from build123d import *

# Parameters (mm, degrees)
SKETCH_1_W      = 36.5
SKETCH_1_H      = 22
EXTRUDE_1_DEPTH = 19
SKETCH_3_R      = 3
EXTRUDE_3_DEPTH = 20
FILLET_1_R      = 5
SKETCH_4_R      = 9
EXTRUDE_4_DEPTH = 24
FILLET_2_R      = 5


with BuildPart() as part:
    # 草图1 → 凸台-拉伸1 (new body)
    with BuildSketch(Plane(origin=(0, 0, 0), x_dir=(0, 0, -1), z_dir=(1, 0, 0))):
        with Locations((18.25, 11)):
            Rectangle(SKETCH_1_W, SKETCH_1_H)
    extrude(amount=EXTRUDE_1_DEPTH)

    # 草图3 → 凸台-拉伸3 (add, symmetric)
    with BuildSketch(Plane(origin=(9.5, 0, 0), x_dir=(0, 0, -1), z_dir=(1, 0, 0))):
        with Locations((25.5, 11)):
            Circle(SKETCH_3_R)
    extrude(amount=EXTRUDE_3_DEPTH, both=True)

    # 圆角1
    fillet_1_edges = [part.edges().sort_by_distance(p)[0] for p in [
        (9.5, 22, -36.5),
        (9.5, 0, -36.5),
    ]]
    fillet(fillet_1_edges, radius=FILLET_1_R)

    # 草图4 → 凸台-拉伸4 (add)
    with BuildSketch(Plane.XY):
        with Locations((9.5, 11.405533056)):
            Circle(SKETCH_4_R)
    extrude(amount=EXTRUDE_4_DEPTH)

    # 圆角2
    fillet_2_edges = [part.edges().sort_by_distance(p)[0] for p in [
        (0.5, 11.405533056, 24),
    ]]
    fillet(fillet_2_edges, radius=FILLET_2_R)


solid = part.part
Design review of the part built by this model. Coordinates are the model's own, in mm. A direction names the side the tool comes from. Round coordinates to 2 decimals unless told otherwise and drop trailing zeros. Loops run counter-clockwise (first coordinate to the right, second up) from the corner with the lowest first, then second, coordinate; pieces in that order, holes last. Notation, with made-up numbers: (41.25, 82.25) - (47.25, 82.25) arc R22 ccw to (47.25, 112.25) - close; hole circle Ø1 at (74, -14.5). An arc over 180 degrees is marked (long way). One line per item, written item: value. Start each with the question number.
1) Consider section B-B on x = 25. Give the boundary of the cut face in (y, z).
2) Draft analysis for pull direction X (two halves, no side actions). For faces 1 (the flat face through (29.5, 11, -25)), 2 (the flat face through (-10.5, 11, -25)), 3 (the cylindrical face through (14.338, 18.994, 9.367)), 4 (the flat face through (9, 11, -36.5)), state which applies: +X half, -X half, draft (parallel to the pull), parting line (faces both ways), or undercut.
3) Insertion check: pin 1 Ø8 at (x, z) = (17.5, 7) entering from -Y; pin 2 Ø1 at (y, z) = (4.5, -7) entering from +X; pin 3 Ø4 at (y, z) = (7, 18) entering from +X. Each pin has a flat end and moves straight along its axis. Give the tip position at first contact, or say it passes through.
4) Consider section C-C on z = -15. Give the boundary of the cut face in (x, y), then the cut area to 3 significant figures.
5) To check wall thickness, follow L1, parallel to X at y = 17.75, z = -7.5; L2, parallel to Z at x = -1, y = 10.75; L3, parallel to Z at x = 8, y = 7.5. State the ranges of each line that lie inside material, in increasing order. Write a range as from..to.
6) Consider section A-A on z = -25.5. Give the boundary of the cut face in (x, y), then the cut area to 3 significant figures.
7) For faces 5 (the cylindrical face through (24.3, 11.1, -22.5)), 6 (the cylindrical face through (-5.2, 11.1, -22.5)), 7 (the cylindrical face through (9.63, 1.43, -35)), 8 (the flat face through (1, 8, 0)), list the 3-axis set-ups (+Z, -Z, +X, -X, +Y, -Y) from which the entire face can be reached by the end or side of a thin tool; tool diameter is ignored.
Reported:
1. outline: circle Ø6 at (11, -25.5)
2. face 1: +X half
2. face 2: -X half
2. face 3: parting line
2. face 4: draft
3. pin 1: stops at y = 3.34
3. pin 2: stops at x = 19
3. pin 3: stops at x = 18.17
4. outline: (0, 0) - (19, 0) - (19, 22) - (0, 22) - close
4. area: 418 mm^2
5. L1: x = 0..19
5. L2: z = -28.49..-22.51
5. L3: z = -36.5..24
6. outline: (-10.5, 8) - (0, 8) - (0, 0) - (19, 0) - (19, 8) - (29.5, 8) - (29.5, 14) - (19, 14) - (19, 22) - (0, 22) - (0, 14) - (-10.5, 14) - close
6. area: 544 mm^2
7. face 5: +X
7. face 6: -X
7. face 7: -Z, +X, -X, -Y
7. face 8: +Z
